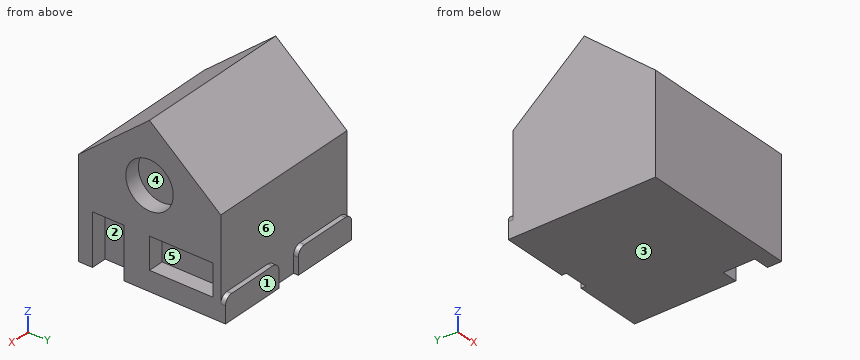
```python
from build123d import *

# Parameters (mm, degrees)
F0_W     = 22.86
F0_H     = 15.864736
F1_DEPTH = 12.7
F2_W     = 5.08
F2_H     = 8.253078
F2_W_2   = 10.16
F2_H_2   = 5.08
F2_R     = 3.81
F3_DEPTH = 2.54
F5_DEPTH = 0.762


with BuildPart() as f1:
    # F0 (on Right) → F1 (new body, symmetric)
    with BuildSketch(Plane.YZ):
        Polygon((0, 17.146922), (-11.43, 7.611658), (11.43, 7.611658), align=None)
        with Locations((0, -0.32071)):
            Rectangle(F0_W, F0_H)
    extrude(amount=F1_DEPTH, both=True)

    # F2 (on face) → F3 (cut)
    with BuildSketch(Plane.YZ.offset(12.7)):
        with Locations((-6.611706, -4.126539)):
            Rectangle(F2_W, F2_H)
        with Locations((5.08, -2.54)):
            Rectangle(F2_W_2, F2_H_2)
        with Locations((0, 7.521919)):
            Circle(F2_R)
    extrude(amount=-F3_DEPTH, mode=Mode.SUBTRACT)

    # F4 (on face) → F5 (join)
    with BuildSketch(Plane(origin=(0, 11.43, 0), x_dir=(-1, 0, 0), z_dir=(0, 1, 0))):
        with BuildLine():
            Line((-5.059074, -4.322298), (-11.43, -4.322298))
            ThreePointArc((-11.43, -4.322298), (-12.328026, -4.694272), (-12.7, -5.592298))
            Line((-12.7, -5.592298), (-12.7, -8.253078))
            Line((-12.7, -8.253078), (-6.329074, -8.253078))
            Line((-6.329074, -8.253078), (-6.329074, -5.592298))
            ThreePointArc((-6.329074, -5.592298), (-5.9571, -4.694272), (-5.059074, -4.322298))
        make_face()
        with BuildLine():
            Line((-3.246726, -4.322298), (-5.059074, -4.322298))
            ThreePointArc((-5.059074, -4.322298), (-5.9571, -4.694272), (-6.329074, -5.592298))
            Line((-6.329074, -5.592298), (-6.329074, -8.253078))
            Line((-6.329074, -8.253078), (-1.976726, -8.253078))
            Line((-1.976726, -8.253078), (-1.976726, -5.592298))
            ThreePointArc((-1.976726, -5.592298), (-2.3487, -4.694272), (-3.246726, -4.322298))
        make_face()
        with BuildLine():
            Line((-3.2258, -4.322298), (-3.246726, -4.322298))
            ThreePointArc((-3.246726, -4.322298), (-2.3487, -4.694272), (-1.976726, -5.592298))
            Line((-1.976726, -5.592298), (-1.976726, -8.253078))
            Line((-1.976726, -8.253078), (-1.9558, -8.253078))
            Line((-1.9558, -8.253078), (-1.9558, -5.592298))
            ThreePointArc((-1.9558, -5.592298), (-2.327774, -4.694272), (-3.2258, -4.322298))
        make_face()
        with BuildLine():
            Line((3.246726, -4.322298), (3.2258, -4.322298))
            ThreePointArc((3.2258, -4.322298), (2.327774, -4.694272), (1.9558, -5.592298))
            Line((1.9558, -5.592298), (1.9558, -8.253078))
            Line((1.9558, -8.253078), (1.976726, -8.253078))
            Line((1.976726, -8.253078), (1.976726, -5.592298))
            ThreePointArc((1.976726, -5.592298), (2.3487, -4.694272), (3.246726, -4.322298))
        make_face()
        with BuildLine():
            Line((5.059074, -4.322298), (3.246726, -4.322298))
            ThreePointArc((3.246726, -4.322298), (2.3487, -4.694272), (1.976726, -5.592298))
            Line((1.976726, -5.592298), (1.976726, -8.253078))
            Line((1.976726, -8.253078), (6.329074, -8.253078))
            Line((6.329074, -8.253078), (6.329074, -5.592298))
            ThreePointArc((6.329074, -5.592298), (5.9571, -4.694272), (5.059074, -4.322298))
        make_face()
        with BuildLine():
            Line((11.43, -4.322298), (5.059074, -4.322298))
            ThreePointArc((5.059074, -4.322298), (5.9571, -4.694272), (6.329074, -5.592298))
            Line((6.329074, -5.592298), (6.329074, -8.253078))
            Line((6.329074, -8.253078), (12.7, -8.253078))
            Line((12.7, -8.253078), (12.7, -5.592298))
            ThreePointArc((12.7, -5.592298), (12.328026, -4.694272), (11.43, -4.322298))
        make_face()
    extrude(amount=F5_DEPTH)


solid = f1.part
```
Design review of the part built by this model. Coordinates are the model's own, in mm. Face numbers are marked on the shaded views. A direction names the side the tool comes from. Coordinates: 2 decimals unless noted, no trailing zeros. Write each loop counter-clockwise with the first axis right and the second up, starting at its lowest first coordinate (ties: lowest second). Pieces come first, ordered by that corner, then holes. Notation, with made-up numbers: M 21.25,87 L 70.25,87 A17 cw 70.25,96 Z; hole C 21,-10.5 d7. An arc over 180 degrees is marked long. Answer as a JSON object with one key per item and string values.
Item 1: Add section A-A, the plane x = -7. Give the boundary of the cut face in (y, z), and give its area (3 significant figures).
Outcome:
{"outline": "M -11.43,-8.25 L 12.19,-8.25 L 12.19,-4.32 L 11.43,-4.32 L 11.43,7.61 L 0,17.15 L -11.43,7.61 Z", "area": "475 mm²"}
Item 2: Add section B-B, the plane z = -3.75. Give the boundary of the cut face in (x, y), and give its area (3 significant figures).
Outcome:
{"outline": "M -12.7,-11.43 L 12.7,-11.43 L 12.7,-9.15 L 10.16,-9.15 L 10.16,-4.07 L 12.7,-4.07 L 12.7,0 L 10.16,0 L 10.16,10.16 L 12.7,10.16 L 12.7,11.43 L -12.7,11.43 Z", "area": "542 mm²"}
Item 3: Draft analysis for pull direction Z (two halves, no side actions). For the marked faces 3, 4, 5 and 6, state which applies: pulls with the +Z half, pulls with the -Z half, needs draft (parallel to the pull), parting line crosses it, or undercut.
Outcome:
{"face 3": "pulls with the -Z half", "face 4": "undercut", "face 5": "undercut", "face 6": "needs draft"}
Item 4: Wall thickness on probe 1 along Z at (x, y) = (11.25, 0.75); probe 2 along X at (y, z) = (5.75, -0.5); probe 3 along Y at (x, z) = (-9.5, 6): over which ranges is each line inside the solid? List them lowest first.
Outcome:
{"probe 1": "-8.25 to -5.08, 0 to 3.79, 11.26 to 16.52", "probe 2": "-12.7 to 10.16", "probe 3": "-11.43 to 11.43"}
Item 5: Machinability: for the marked faces 1 and 2, which of the approach directions +Z, -Z, +X, -X, +Y, -Y give a long, thin tool a straight path to every point of the face, cutting with its end or side? Answer none if there is none.
Outcome:
{"face 1": "+Z, -Z, +X, -X, +Y", "face 2": "-Z, +X"}
Item 6: Add section C-C, the plane y = -0.5. Give the boundary of the cut face in (x, z).
Outcome:
{"outline": "M -12.7,-8.25 L 12.7,-8.25 L 12.7,3.74 L 10.16,3.74 L 10.16,11.3 L 12.7,11.3 L 12.7,16.73 L -12.7,16.73 Z"}
Item 7: Insertion check: pin 1 Ø5 at (x, z) = (-5, -1) entering from +Y; pin 2 Ø1.5 at (y, z) = (3, -3) entering from +X; pin 3 Ø0.8 at (x, y) = (11.5, 6.5) entering from +Z. Each pin has a flat end and moves straight along its axis. Give the tip position at first contact, or say it passes through.
Outcome:
{"pin 1": "y = 11.43", "pin 2": "x = 10.16", "pin 3": "z = 12.06"}
Item 8: Add section D-D, the plane z = 5.75. Give the boundary of the cut face in (x, y).
Outcome:
{"outline": "M -12.7,-11.43 L 12.7,-11.43 L 12.7,-3.37 L 10.16,-3.37 L 10.16,3.37 L 12.7,3.37 L 12.7,11.43 L -12.7,11.43 Z"}
